Could you check a few things on this model? Use its own coordinates, in mm. Give positions to 0.01 mm unless a question says otherwise; leave off trailing zeros. Use one line per item in the form item = value.
from build123d import *

# Parameters (mm, degrees)
SKETCH3_W           = 210
SKETCH3_H           = 50
BOSS_EXTRUDE1_DEPTH = 5
SKETCH8_R           = 1.5
CUT_EXTRUDE1_DEPTH  = 5


with BuildPart() as part:
    # Sketch3 → Boss-Extrude1 (new body)
    with BuildSketch(Plane.XY):
        Polygon((-265, -25), (-105, -25), (-105, 25), (-265, 15), align=None)
        with BuildLine():
            Line((-275, -25), (-265, -25))
            Line((-265, -25), (-265, 15))
            ThreePointArc((-265, 15), (-284.634416342, -1.341395914), (-275, -25))
        make_face()
        Rectangle(SKETCH3_W, SKETCH3_H)
        Polygon((105, 25), (105, -25), (265, -25), (265, 15), align=None)
        with BuildLine():
            Line((265, 15), (265, -25))
            Line((265, -25), (275, -25))
            ThreePointArc((275, -25), (284.634416342, -1.341395914), (265, 15))
        make_face()
    extrude(amount=BOSS_EXTRUDE1_DEPTH)

    # Sketch8 → Cut-Extrude1 (cut)
    with BuildSketch(Plane.XY.offset(5)):
        with Locations((0, 11)):
            Circle(SKETCH8_R)
        with Locations((0, 1)):
            Circle(SKETCH8_R)
        with Locations((0, -9)):
            Circle(SKETCH8_R)
        with Locations((0, -19)):
            Circle(SKETCH8_R)
        with Locations((50.8, 11)):
            Circle(SKETCH8_R)
        with Locations((50.8, -9)):
            Circle(SKETCH8_R)
        with Locations((50.8, 1)):
            Circle(SKETCH8_R)
        with Locations((50.8, -19)):
            Circle(SKETCH8_R)
        with Locations((101.6, 11)):
            Circle(SKETCH8_R)
        with Locations((101.6, -9)):
            Circle(SKETCH8_R)
        with Locations((101.6, 1)):
            Circle(SKETCH8_R)
        with Locations((101.6, -19)):
            Circle(SKETCH8_R)
        with Locations((-50.8, 11)):
            Circle(SKETCH8_R)
        with Locations((-50.8, 1)):
            Circle(SKETCH8_R)
        with Locations((-50.8, -9)):
            Circle(SKETCH8_R)
        with Locations((-50.8, -19)):
            Circle(SKETCH8_R)
        with Locations((-101.6, 11)):
            Circle(SKETCH8_R)
        with Locations((-101.6, 1)):
            Circle(SKETCH8_R)
        with Locations((-101.6, -9)):
            Circle(SKETCH8_R)
        with Locations((-101.6, -19)):
            Circle(SKETCH8_R)
    extrude(amount=-CUT_EXTRUDE1_DEPTH, mode=Mode.SUBTRACT)


solid = part.part
1) If I drill on L1, parallel to Y at x = 101.6, z = 3.7; L2, parallel to X at y = 0.5, z = 4; L3, parallel to X at y = -6, z = 3.65, over which ranges is the centre line in solid material (lowest first)?
Checked values:
L1 = -25 to -20.5, -17.5 to -10.5, -7.5 to -0.5, 2.5 to 9.5, 12.5 to 25
L2 = -284.09 to -103.01, -100.19 to -52.21, -49.39 to -1.41, 1.41 to 49.39, 52.21 to 100.19, 103.01 to 284.09
L3 = -285.27 to 285.27
2) I want a section at A-A, the plane z = 3.8. Count the separate pieces of the cut face and the enclosed holes in it, plus the area to 3 significant figures.
Checked values:
separate_pieces = 1
enclosed_holes = 20
area = 26,100 mm2
3) For pin 1 Ø1.8 at (x, y) = (-101.6, -19) entering from +Z; pin 2 Ø2 at (x, z) = (-166.5, 2) entering from +Y; pin 3 Ø1 at (x, z) = (182, 4) entering from +Y, each with a flat end and sliding along its axis, tell me the tip position at first contact or that it passes through.
Checked values:
pin_1 = through
pin_2 = 21.22
pin_3 = 20.22
